Check sheet for the modelled part. Datum: model origin and axes. Units: mm. A direction names the side the tool comes from. Round coordinates to 2 decimals unless told otherwise and drop trailing zeros. Loops run counter-clockwise (first coordinate to the right, second up) from the corner with the lowest first, then second, coordinate; pieces in that order, holes last. Notation, with made-up numbers: (58.25, -9.75) - (84.25, -9.75) arc R5 ccw to (84.25, -4.75) - close; hole circle Ø10 at (70, 43.5). An arc over 180 degrees is marked (long way). Answer in a Markdown table with one row per item. Add a question column.
(1) Cross-section at C-C on z = -17. Enter the section's corners in (x, y).
(2) Access from +Z, -Z, +X, -X, +Y, -Y to the whole of each face (thin tool, end or side, straight path). Record for faces 1 (the flat face through (1, 14, -10.795)), 2 (the flat face through (38.1, 19, -13)), 3 (the flat face through (19, 16, -19.05)).
(3) Cross-section at A-A on y = 8. Enter the section's corners in (x, z) (3 decimals), then the cut area to 3 significant figures.
(4) Thickness scan on line 1 along Z through (x, y) = (18, 14.5) (3 decimals); line 2 along X through (y, z) = (18.5, -17.75); line 3 along Z through (x, y) = (13, 30.5) (3 decimals). Record the ranges inside material, lowest first.
(5) Cross-section at B-B on x = 33. Enter the section's corners in (y, z) (3 decimals), then the cut area to 3 significant figures.
(6) Mould release check, pull along Z, two halves, no side actions. Record for faces 4 (the flat face through (19, 0, -1)), 5 (the flat face through (19, 19, 0)), 6 (the flat face through (36.83, 16, -14)): +Z half, -Z half, draft (parallel to the pull), parting line (faces both ways), or undercut.
(7) Cross-section at D-D on z = -3.25. Enter the section's corners in (x, y), then the cut area to 3 significant figures.
(8) Gauge pin test, flat end, axial feed: pin 1 (10 mm diameter, centred on x = 16, z = -11, fed in from -Y). Record the tip position at first contact, or that the pin passes through.
from build123d import *

# Parameters (mm, degrees)
SKETCH1_W           = 38.1
SKETCH1_H           = 22.225
BOSS_EXTRUDE2_DEPTH = 38.1
SKETCH4_W           = 35.56
SKETCH4_H           = 12.7
CUT_EXTRUDE1_DEPTH  = 31.75
SKETCH5_W           = 8.89
SKETCH5_H           = 29.21
CUT_EXTRUDE3_DEPTH  = 59.285252208


with BuildPart() as part:
    # Sketch1 → Boss-Extrude2 (new body)
    with BuildSketch(Plane(origin=(0, 0, 0), x_dir=(1, 0, 0), z_dir=(0, 1, 0))):
        with Locations((19.05, 11.1125)):
            Rectangle(SKETCH1_W, SKETCH1_H)
    extrude(amount=BOSS_EXTRUDE2_DEPTH)

    # Sketch4 → Cut-Extrude1 (cut)
    with BuildSketch(Plane.XZ):
        with Locations((19.05, -12.7)):
            Rectangle(SKETCH4_W, SKETCH4_H)
    extrude(amount=-CUT_EXTRUDE1_DEPTH, mode=Mode.SUBTRACT)

    # Sketch5 → Cut-Extrude3 (cut, through all)
    with BuildSketch(Plane.ZY):
        with Locations((-6.350275286, 14.051077043)):
            Rectangle(SKETCH5_W, SKETCH5_H)
    extrude(amount=-CUT_EXTRUDE3_DEPTH, mode=Mode.SUBTRACT)


solid = part.part
Answers:
| question | item | result |
|---|---|---|
| 1 | outline | (0, 0) - (1.27, 0) - (1.27, 31.75) - (36.83, 31.75) - (36.83, 0) - (38.1, 0) - (38.1, 38.1) - (0, 38.1) - close |
| 2 | face 1 | +X, -X, -Y |
| 2 | face 2 | +Z, -Z, +X, +Y, -Y |
| 2 | face 3 | -Y |
| 3 | outline | (0, -22.225) - (38.1, -22.225) - (38.1, -10.795) - (36.83, -10.795) - (36.83, -19.05) - (1.27, -19.05) - (1.27, -10.795) - (0, -10.795) - close; (0, -1.905) - (38.1, -1.905) - (38.1, 0) - (0, 0) - close |
| 3 | area | 215 mm^2 |
| 4 | line 1 | z = -22.225 to -19.05, -1.905 to 0 |
| 4 | line 2 | x = 0 to 1.27, 36.83 to 38.1 |
| 4 | line 3 | z = -22.225 to -19.05, -6.35 to 0 |
| 5 | outline | (0, -22.225) - (38.1, -22.225) - (38.1, 0) - (0, 0) - (0, -1.905) - (28.656, -1.905) - (28.656, -6.35) - (31.75, -6.35) - (31.75, -19.05) - (0, -19.05) - close |
| 5 | area | 316 mm^2 |
| 6 | face 4 | draft |
| 6 | face 5 | +Z half |
| 6 | face 6 | undercut |
| 7 | outline | (0, 28.66) - (38.1, 28.66) - (38.1, 38.1) - (0, 38.1) - close |
| 7 | area | 360 mm^2 |
| 8 | pin 1 | stops at y = 28.66 |
